Build history of the part. All positions in model axes, mm. A direction names the side the tool comes from. Give positions to 0.01 mm unless a question says otherwise; leave off trailing zeros. Order: outer loops, then holes, each group sorted by start corner. A loop starts at its lowest first (then second) coordinate and runs counter-clockwise, first axis right, second up. Notation, with made-up numbers: (39.25, -40) -> (43.25, -40) arc R12 ccw to (43.25, -29) -> close; hole circle Ø2 at (33.5, 8). An arc over 180 degrees is marked (long way). One line per item, written item: value. Start each with the question number.
(1) Saw through at A-A on z = 5.5. Give the cut face in (x, y), plus the area to 3 significant figures.
(2) Saw through at B-B on x = 4.5. Give the cut face in (y, z).
(3) Saw through at C-C on x = -2. Give the cut face in (y, z).
(4) Saw through at D-D on z = 2.75. Give the cut face in (x, y).
(5) Probe line 1 (Z direction, x = 7.5, y = 0.3); line 2 (X direction, y = 0.1, z = 0); line 3 (Z direction, x = 1, y = 0.4). List the from-to ranges inside material, lowest first.
(6) Two-plate mould, pull along X, no slides. Class faces 1 (the flat face through (1, 0, 0)), 2 (the flat face through (-2.68, 0.25, -1.48)), 3 (the flat face through (9.462, 0.247, 6.793)): +X half, -X half, draft (parallel to the pull), parting line (faces both ways), or undercut.
(7) Which spindle directions (+Z, -Z, +X, -X, +Y, -Y) get a long thin tool onto all of the face, cutting with end or side? Do faces 4 (the flat face through (-0.67, 0.25, 1.48)), 5 (the flat face through (9.448, 0.246, -6.807)). Say none if no direction does.
```python
from build123d import *

# Parameters (mm, degrees)
SKETCH1_W           = 2
SKETCH1_H           = 1.8
BOSS_EXTRUDE1_DEPTH = 0.5
CHAMFER1_SIZE       = 0.2


with BuildPart() as part:
    # Sketch1 → Boss-Extrude1 (new body)
    with BuildSketch(Plane(origin=(0, 0, 0), x_dir=(1, 0, 0), z_dir=(0, 1, 0))):
        with BuildLine():
            Line((-6.744590168, 7.3), (8.955409832, 7.3))
            Line((8.955409832, 7.3), (9.955409832, 6.3))
            Line((9.955409832, 6.3), (9.955409832, 2.3))
            Line((9.955409832, 2.3), (4.955409832, 2.3))
            Line((4.955409832, 2.3), (4.955409832, 2.5))
            Line((4.955409832, 2.5), (-1.565729119, 2.5))
            Line((-1.565729119, 2.5), (-3.83310718, 0.421156991))
            ThreePointArc((-3.83310718, 0.421156991), (-3.912248176, -0.508574312), (-2.992299199, -0.664643125))
            Line((-2.992299199, -0.664643125), (-2.267378061, 0))
            Line((-2.267378061, 0), (-0.859569395, 1.290747782))
            ThreePointArc((-0.859569395, 1.290747782), (1.169124512, 1.029390936), (1.022775524, -1.010826784))
            Line((1.022775524, -1.010826784), (0.345859604, -1.63145638))
            ThreePointArc((0.345859604, -1.63145638), (0.216903786, -2.179100893), (0.679037836, -2.5))
            Line((0.679037836, -2.5), (4.955409832, -2.5))
            Line((4.955409832, -2.5), (4.955409832, -2.3))
            Line((4.955409832, -2.3), (9.955409832, -2.3))
            Line((9.955409832, -2.3), (9.955409832, -6.3))
            Line((9.955409832, -6.3), (8.955409832, -7.3))
            Line((8.955409832, -7.3), (-6.744590168, -7.3))
            Line((-6.744590168, -7.3), (-6.744590168, -6.153555701))
            Line((-6.744590168, -6.153555701), (-7.744590168, -6.153555701))
            Line((-7.744590168, -6.153555701), (-7.744590168, -4.753555701))
            Line((-7.744590168, -4.753555701), (-5.644590168, -4.753555701))
            Line((-5.644590168, -4.753555701), (-5.644590168, -2.5))
            Line((-5.644590168, -2.5), (-1.785240618, -2.5))
            Line((-1.785240618, -2.5), (0.482137442, -0.421156991))
            ThreePointArc((0.482137442, -0.421156991), (0.561278438, 0.508574312), (-0.358670538, 0.664643125))
            Line((-0.358670538, 0.664643125), (-1.083591677, 0))
            Line((-1.083591677, 0), (-2.491400342, -1.290747782))
            ThreePointArc((-2.491400342, -1.290747782), (-4.52009425, -1.029390936), (-4.373745262, 1.010826784))
            Line((-4.373745262, 1.010826784), (-3.696829341, 1.63145638))
            ThreePointArc((-3.696829341, 1.63145638), (-3.568749704, 2.181284569), (-4.034728143, 2.5))
            Line((-4.034728143, 2.5), (-5.644590168, 2.5))
            Line((-5.644590168, 2.5), (-5.644590168, 4.753555701))
            Line((-5.644590168, 4.753555701), (-7.744590168, 4.753555701))
            Line((-7.744590168, 4.753555701), (-7.744590168, 6.153555701))
            Line((-7.744590168, 6.153555701), (-6.744590168, 6.153555701))
            Line((-6.744590168, 6.153555701), (-6.744590168, 7.3))
        make_face()
        with Locations((-0.244590168, 5.7)):
            Rectangle(SKETCH1_W, SKETCH1_H, mode=Mode.SUBTRACT)
        with Locations((-0.244590168, -5.7)):
            Rectangle(SKETCH1_W, SKETCH1_H, mode=Mode.SUBTRACT)
    extrude(amount=BOSS_EXTRUDE1_DEPTH)

    # Chamfer1
    chamfer1_edges = [part.edges().sort_by_distance(p)[0] for p in [
        (9.955409832, 0.5, -4.3),
        (9.955409832, 0, -4.3),
        (9.955409832, 0, 4.3),
        (9.955409832, 0.5, 4.3),
    ]]
    chamfer(chamfer1_edges, length=CHAMFER1_SIZE)


solid = part.part
```
Results below:
1. outline: (-7.74, 0) -> (-1.24, 0) -> (-1.24, 0.5) -> (-7.74, 0.5) -> close; (0.76, 0) -> (9.76, 0) -> (9.96, 0.2) -> (9.96, 0.3) -> (9.76, 0.5) -> (0.76, 0.5) -> close
1. area: 7.81 mm²
2. outline: (0, -7.3) -> (0.5, -7.3) -> (0.5, -2.5) -> (0, -2.5) -> close; (0, 2.5) -> (0.5, 2.5) -> (0.5, 7.3) -> (0, 7.3) -> close
3. outline: (0, -7.3) -> (0.5, -7.3) -> (0.5, -2.1) -> (0, -2.1) -> close; (0, -0.25) -> (0.5, -0.25) -> (0.5, 0.84) -> (0, 0.84) -> close; (0, 2.5) -> (0.5, 2.5) -> (0.5, 7.3) -> (0, 7.3) -> close
4. outline: (-5.64, 0) -> (9.76, 0) -> (9.96, 0.2) -> (9.96, 0.3) -> (9.76, 0.5) -> (-5.64, 0.5) -> close
5. line 1: z = -7.3 to -2.3, 2.3 to 7.3
5. line 2: x = -4.85 to -4.05, -2.27 to -1.08, 0.7 to 1.5
5. line 3: z = -7.3 to -2.5, -1.2 to 1.03, 2.5 to 7.3
6. face 1: draft
6. face 2: undercut
6. face 3: +X half
7. face 4: +Y, -Y
7. face 5: -Z, +X, +Y, -Y
